from build123d import *

# Parameters (mm, degrees)
BOSS_EXTRUDE1_DEPTH = 25.4
SKETCH2_R           = 1.5
CUT_EXTRUDE1_DEPTH  = 120.2689793


with BuildPart() as part:
    # Sketch1 → Boss-Extrude1 (new body)
    with BuildSketch(Plane(origin=(0, 0, 0), x_dir=(1, 0, 0), z_dir=(0, 1, 0))):
        Polygon((-21.143554781, 20.976139754), (-21.143554781, -21.178999859), (-15.143554781, -21.178999859), (-15.143554781, -18.178999859), (-18.143554781, -18.178999859), (-18.143554781, 19.921000141), (-19.143705232, 18.939106358), align=None)
        Polygon((16.956445219, -18.178999859), (16.956445219, -21.178999859), (22.956445219, -21.178999859), (22.956445219, 20.976139754), (20.956595671, 18.939106358), (19.956445219, 19.921000141), (19.956445219, -18.178999859), align=None)
        Polygon((-18.000706286, 20.061241092), (-18.143554781, 19.921000141), (-17.629307024, 19.921000141), align=None)
        Polygon((-21.143554781, 23.921000141), (-21.143554781, 20.976139754), (-19.143705232, 18.939106358), (-18.143554781, 19.921000141), (-18.000706286, 20.061241092), (-19.950434941, 20.797461723), (-18.770981881, 23.921000141), align=None)
        Polygon((-18.429197778, 23.921000141), (-18.770981881, 23.921000141), (-19.950434941, 20.797461723), (-18.000706286, 20.061241092), (-16.289346466, 21.741361883), align=None)
        Polygon((-14.495314995, 23.921000141), (-18.429197778, 23.921000141), (-16.289346466, 21.741361883), (-18.000706286, 20.061241092), (-17.629307024, 19.921000141), (-16.005721338, 19.921000141), align=None)
        Polygon((-18.676040592, 24.172432584), (-18.770981881, 23.921000141), (-18.429197778, 23.921000141), align=None)
        Polygon((-67.6732731, 68.371000141), (-21.143554781, 20.976139754), (-21.143554781, 23.921000141), (-18.770981881, 23.921000141), (-18.676040592, 24.172432584), (-62.06781096, 68.371000141), align=None)
        Polygon((-18.676040592, 24.172432584), (-18.429197778, 23.921000141), (-14.495314995, 23.921000141), (0.906445219, 64.70938874), (-0.476185052, 68.371000141), (-1.986591395, 68.371000141), align=None)
        Polygon((16.308205433, 23.921000141), (-14.495314995, 23.921000141), (-16.005721338, 19.921000141), (17.818611776, 19.921000141), align=None)
        Polygon((17.818611776, 19.921000141), (19.442197463, 19.921000141), (19.813596724, 20.061241092), (18.102236904, 21.741361883), (20.242088216, 23.921000141), (16.308205433, 23.921000141), align=None)
        Polygon((21.763325379, 20.797461723), (20.583872319, 23.921000141), (20.242088216, 23.921000141), (18.102236904, 21.741361883), (19.813596724, 20.061241092), align=None)
        Polygon((20.956595671, 18.939106358), (22.956445219, 20.976139754), (22.956445219, 23.921000141), (20.583872319, 23.921000141), (21.763325379, 20.797461723), (19.813596724, 20.061241092), (19.956445219, 19.921000141), align=None)
        Polygon((19.442197463, 19.921000141), (19.956445219, 19.921000141), (19.813596724, 20.061241092), align=None)
        Polygon((0.906445219, 64.70938874), (16.308205433, 23.921000141), (20.242088216, 23.921000141), (20.48893103, 24.172432584), (3.799481834, 68.371000141), (2.289075491, 68.371000141), align=None)
        Polygon((22.956445219, 23.921000141), (22.956445219, 20.976139754), (69.486163538, 68.371000141), (63.880701399, 68.371000141), (20.48893103, 24.172432584), (20.583872319, 23.921000141), align=None)
        Polygon((63.880701399, 68.371000141), (69.486163538, 68.371000141), (66.631804771, 71.173255667), align=None)
        Polygon((-67.6732731, 72.371000141), (-67.6732731, 68.371000141), (-64.818914333, 71.173255667), (-62.06781096, 68.371000141), (-1.986591395, 68.371000141), (-1.35741728, 70.037238153), (0.906445219, 69.182400084), (3.170307718, 70.037238153), (3.799481834, 68.371000141), (63.880701399, 68.371000141), (66.631804771, 71.173255667), (69.486163538, 68.371000141), (69.486163538, 72.371000141), align=None)
        Polygon((2.289075491, 68.371000141), (-0.476185052, 68.371000141), (0.906445219, 64.70938874), align=None)
        Polygon((-1.35741728, 70.037238153), (-1.986591395, 68.371000141), (-0.476185052, 68.371000141), (-0.571798584, 68.62421288), (0.906445219, 69.182400084), align=None)
        Polygon((-0.571798584, 68.62421288), (-0.476185052, 68.371000141), (2.289075491, 68.371000141), (2.384689022, 68.62421288), (0.906445219, 69.182400084), align=None)
        Polygon((2.384689022, 68.62421288), (2.289075491, 68.371000141), (3.799481834, 68.371000141), (3.170307718, 70.037238153), (0.906445219, 69.182400084), align=None)
        Polygon((-64.818914333, 71.173255667), (-67.6732731, 68.371000141), (-62.06781096, 68.371000141), align=None)
        Polygon((20.242088216, 23.921000141), (20.583872319, 23.921000141), (20.48893103, 24.172432584), align=None)
    extrude(amount=BOSS_EXTRUDE1_DEPTH)

    # Sketch2 → Cut-Extrude1 (cut, through all)
    with BuildSketch(Plane(origin=(0, 0, -72.371000141), x_dir=(-1, 0, 0), z_dir=(0, 0, -1))):
        with Locations((37.6732731, 6.7)):
            Circle(SKETCH2_R)
        with Locations((37.6732731, 18.7)):
            Circle(SKETCH2_R)
        with Locations((-39.486163538, 18.7)):
            Circle(SKETCH2_R)
        with Locations((-39.486163538, 6.7)):
            Circle(SKETCH2_R)
    extrude(amount=-CUT_EXTRUDE1_DEPTH, mode=Mode.SUBTRACT)


solid = part.part
Design review of the part built by this model. Coordinates are the model's own, in mm. A direction names the side the tool comes from. Give positions to 0.01 mm unless a question says otherwise; leave off trailing zeros. Write each loop counter-clockwise with the first axis right and the second up, starting at its lowest first coordinate (ties: lowest second). Pieces come first, ordered by that corner, then holes. Notation, with made-up numbers: M -32,63 L -8,63 A17 cw -8,89 Z; hole C 77,-21 d11. An arc over 180 degrees is marked long. Answer as a JSON object with one key per item and string values. Group by question number.
1) Tool access review of faces 1 (the face through (-15.144, 13, 20)), 2 (the face through (2, 13, -72.371)), 3 (the face through (-6.9, 12.52, -44.03)): name each direction out of +Z, -Z, +X, -X, +Y, -Y from which nothing blocks a thin tool from reaching the whole face with its end or side.
2) We need section B-B (x = 31). Give the boundary of the cut face in (y, z), and give its area (3 significant figures).
3) For line 1 along X through (y, z) = (22, -52); line 2 along X through (y, z) = (6.7, -38); line 3 along X through (y, z) = (21.75, 7), list the stretches that pass through material, from the lowest coordinate up.
4) We need section A-A (y = 22). Give the boundary of the cut face in (x, z).
5) We need section C-C (z = -49). Give the boundary of the cut face in (x, y).
6) Clearance check with flat-ended pins moving along their axes: pin 1 Ø2.5 at (y, z) = (14.5, 20) entering from +X; pin 2 Ø6 at (y, z) = (9.5, -62.5) entering from +X; pin 3 Ø3.5 at (x, y) = (-37.67, 6.7) entering from +Z. State where each tip first meets the part, or that it passes through.
7) Mouldability with a two-part tool opening along Z and no side actions: class faces 4 (the face through (-18, 13, 21.179)), 5 (the face through (18, 13, 18.179)), 6 (the face through (1, 13, -23.921)), 7 (the face through (38.79, 17.37, -40.8)) as released by +Z, released by -Z, zero draft, split by the parting line, or undercut.
Answer key:
{
 "1": {"face 1": "+Z, +Y, -Y", "face 2": "-Z, +X, -X, +Y, -Y", "face 3": "+Y, -Y"},
 "2": {"outline": "M 0,-72.37 L 25.4,-72.37 L 25.4,-68.37 L 0,-68.37 Z; M 0,-34.88 L 25.4,-34.88 L 25.4,-29.17 L 0,-29.17 Z", "area": "247 mm²"},
 "3": {"line 1": "x = -51.6 to -46, -8.17 to -3.89, 5.71 to 9.98, 47.81 to 53.41", "line 2": "x = -36.17 to -32.25, -13.45 to -9.18, 10.99 to 15.27, 34.06 to 37.99", "line 3": "x = -21.14 to -18.14, 19.96 to 22.96"},
 "4": {"outline": "M -67.67,-72.37 L 69.49,-72.37 L 69.49,-68.37 L 22.96,-20.98 L 22.96,21.18 L 16.96,21.18 L 16.96,18.18 L 19.96,18.18 L 19.96,-19.92 L -18.14,-19.92 L -18.14,18.18 L -15.14,18.18 L -15.14,21.18 L -21.14,21.18 L -21.14,-20.98 L -67.67,-68.37 Z; hole M -62.07,-68.37 L -1.99,-68.37 L -18.68,-24.17 Z; hole M -14.5,-23.92 L 0.91,-64.71 L 16.31,-23.92 Z; hole M 3.8,-68.37 L 63.88,-68.37 L 20.49,-24.17 Z"},
 "5": {"outline": "M -48.66,0 L -43.05,0 L -43.05,25.4 L -48.66,25.4 Z; M -9.3,0 L -5.03,0 L -5.03,25.4 L -9.3,25.4 Z; M 6.84,0 L 11.11,0 L 11.11,25.4 L 6.84,25.4 Z; M 44.86,0 L 50.47,0 L 50.47,25.4 L 44.86,25.4 Z"},
 "6": {"pin 1": "stops at x = 22.96", "pin 2": "stops at x = 66.67", "pin 3": "stops at z = -36.03"},
 "7": {"face 4": "released by +Z", "face 5": "undercut", "face 6": "undercut", "face 7": "zero draft"}
}
